from build123d import *

# Parameters (mm, degrees)
BOSS_EXTRUDE1_DEPTH = 15
CUT_EXTRUDE1_DEPTH  = 1.5
SKETCH3_R           = 1.75
CUT_EXTRUDE2_DEPTH  = 9.5
SKETCH5_W           = 31
SKETCH5_H           = 4
CUT_EXTRUDE3_DEPTH  = 54.5
SKETCH9_R           = 5.75
CUT_EXTRUDE6_DEPTH  = 30
CUT_EXTRUDE7_DEPTH  = 1
CUT_EXTRUDE8_DEPTH  = 36


with BuildPart() as part:
    # Sketch1 → Boss-Extrude1 (new body)
    with BuildSketch(Plane.XY):
        with BuildLine():
            Line((0, 20), (40, 20))
            Line((40, 20), (40, -20))
            Line((40, -20), (0, -20))
            ThreePointArc((0, -20), (-20, 0), (0, 20))
        make_face()
    extrude(amount=BOSS_EXTRUDE1_DEPTH)

    # Sketch2 → Cut-Extrude1 (cut)
    with BuildSketch(Plane.XY.offset(15)):
        Polygon((0, 3.58), (-3.100370946, 1.79), (-3.100370946, -1.79), (0, -3.58), (3.100370946, -1.79), (3.100370946, 1.79), align=None)
    cut_extrude1 = extrude(amount=-CUT_EXTRUDE1_DEPTH, mode=Mode.SUBTRACT)

    # Mirror1: Cut-Extrude1 across plane
    add(cut_extrude1.mirror(Plane.XY.offset(7.5)), mode=Mode.SUBTRACT)

    # Sketch3 → Cut-Extrude2 (cut)
    with BuildSketch(Plane.XY.offset(13.5)):
        Circle(SKETCH3_R)
    extrude(amount=-CUT_EXTRUDE2_DEPTH, mode=Mode.SUBTRACT)

    # Sketch5 → Cut-Extrude3 (cut)
    with BuildSketch(Plane.XZ.offset(20)):
        with Locations((-4.5, 7.5)):
            Rectangle(SKETCH5_W, SKETCH5_H)
    extrude(amount=-CUT_EXTRUDE3_DEPTH, mode=Mode.SUBTRACT)

    # Loft2: read off the stored shape, not the designer's step
    # Loft2: loft between two sections, ruled curve by curve
    loft2_from = [
        Edge.make_bspline([(60, 9.363291776, 3.988765584), (60, 9.089319173, 3.258171977), (60, 8.706678231, 2.497933469), (60, 7.661601681, 1.009485762), (60, 6.997280046, 0.281867871), (60, 5.377038752, -0.99416351), (60, 4.420018042, -1.539958552), (60, 2.836034453, -2.105793102), (60, 2.284258254, -2.252472584), (60, 1.154936709, -2.449606951), (60, 0.57750039, -2.5), (60, -0.57750039, -2.5), (60, -1.154936709, -2.449606951), (60, -2.284258254, -2.252472584), (60, -2.836034453, -2.105793102), (60, -4.420018042, -1.539958552), (60, -5.377038752, -0.99416351), (60, -6.997280046, 0.281867871), (60, -7.661601681, 1.009485762), (60, -8.706678231, 2.497933469), (60, -9.089319173, 3.258171977), (60, -9.363291776, 3.988765584)], [0, 0, 0, 0, 0.125, 0.125, 0.25, 0.25, 0.375, 0.375, 0.4375, 0.4375, 0.5, 0.5, 0.5625, 0.5625, 0.625, 0.625, 0.75, 0.75, 0.875, 0.875, 1, 1, 1, 1], 3),
        Edge.make_bspline([(60, -9.363291776, 3.988765584), (60, -9.568771228, 4.53671079), (60, -9.729102032, 5.111695552), (60, -9.944756725, 6.291183156), (60, -10, 6.895551394), (60, -10, 8.104448606), (60, -9.944756725, 8.708816844), (60, -9.729102032, 9.888304448), (60, -9.568771228, 10.46328921), (60, -9.363291776, 11.011234416)], [0, 0, 0, 0, 0.25, 0.25, 0.5, 0.5, 0.75, 0.75, 1, 1, 1, 1], 3),
        Edge.make_bspline([(60, 9.363291776, 11.011234416), (60, 9.568771228, 10.46328921), (60, 9.729102032, 9.888304448), (60, 9.944756725, 8.708816844), (60, 10, 8.104448606), (60, 10, 6.895551394), (60, 9.944756725, 6.291183156), (60, 9.729102032, 5.111695552), (60, 9.568771228, 4.53671079), (60, 9.363291776, 3.988765584)], [0, 0, 0, 0, 0.25, 0.25, 0.5, 0.5, 0.75, 0.75, 1, 1, 1, 1], 3),
        Edge.make_bspline([(60, -9.363291776, 11.011234416), (60, -9.089319173, 11.741828023), (60, -8.706678231, 12.502066531), (60, -7.661601681, 13.990514238), (60, -6.997280046, 14.718132129), (60, -5.377038752, 15.99416351), (60, -4.420018042, 16.539958552), (60, -2.836034453, 17.105793102), (60, -2.284258254, 17.252472584), (60, -1.154936709, 17.449606951), (60, -0.57750039, 17.5), (60, 0.57750039, 17.5), (60, 1.154936709, 17.449606951), (60, 2.284258254, 17.252472584), (60, 2.836034453, 17.105793102), (60, 4.420018042, 16.539958552), (60, 5.377038752, 15.99416351), (60, 6.997280046, 14.718132129), (60, 7.661601681, 13.990514238), (60, 8.706678231, 12.502066531), (60, 9.089319173, 11.741828023), (60, 9.363291776, 11.011234416)], [0, 0, 0, 0, 0.125, 0.125, 0.25, 0.25, 0.375, 0.375, 0.4375, 0.4375, 0.5, 0.5, 0.5625, 0.5625, 0.625, 0.625, 0.75, 0.75, 0.875, 0.875, 1, 1, 1, 1], 3),
    ]
    loft2_to = [
        Edge.make_bspline([(40, 20, 0), (40, 18.333333333, 0), (40, 16.666666667, 0), (40, 13.333333333, 0), (40, 11.666666667, 0), (40, 8.333333333, 0), (40, 6.666666667, 0), (40, 4.166666667, 0), (40, 3.333333333, 0), (40, 1.666666667, 0), (40, 0.833333333, 0), (40, -0.833333333, 0), (40, -1.666666667, 0), (40, -3.333333333, 0), (40, -4.166666667, 0), (40, -6.666666667, 0), (40, -8.333333333, 0), (40, -11.666666667, 0), (40, -13.333333333, 0), (40, -16.666666667, 0), (40, -18.333333333, 0), (40, -20, 0)], [0, 0, 0, 0, 0.125, 0.125, 0.25, 0.25, 0.375, 0.375, 0.4375, 0.4375, 0.5, 0.5, 0.5625, 0.5625, 0.625, 0.625, 0.75, 0.75, 0.875, 0.875, 1, 1, 1, 1], 3),
        Edge.make_bspline([(40, -20, 0), (40, -20, 1.25), (40, -20, 2.5), (40, -20, 5), (40, -20, 6.25), (40, -20, 8.75), (40, -20, 10), (40, -20, 12.5), (40, -20, 13.75), (40, -20, 15)], [0, 0, 0, 0, 0.25, 0.25, 0.5, 0.5, 0.75, 0.75, 1, 1, 1, 1], 3),
        Edge.make_bspline([(40, 20, 15), (40, 20, 13.75), (40, 20, 12.5), (40, 20, 10), (40, 20, 8.75), (40, 20, 6.25), (40, 20, 5), (40, 20, 2.5), (40, 20, 1.25), (40, 20, 0)], [0, 0, 0, 0, 0.25, 0.25, 0.5, 0.5, 0.75, 0.75, 1, 1, 1, 1], 3),
        Edge.make_bspline([(40, -20, 15), (40, -18.333333333, 15), (40, -16.666666667, 15), (40, -13.333333333, 15), (40, -11.666666667, 15), (40, -8.333333333, 15), (40, -6.666666667, 15), (40, -4.166666667, 15), (40, -3.333333333, 15), (40, -1.666666667, 15), (40, -0.833333333, 15), (40, 0.833333333, 15), (40, 1.666666667, 15), (40, 3.333333333, 15), (40, 4.166666667, 15), (40, 6.666666667, 15), (40, 8.333333333, 15), (40, 11.666666667, 15), (40, 13.333333333, 15), (40, 16.666666667, 15), (40, 18.333333333, 15), (40, 20, 15)], [0, 0, 0, 0, 0.125, 0.125, 0.25, 0.25, 0.375, 0.375, 0.4375, 0.4375, 0.5, 0.5, 0.5625, 0.5625, 0.625, 0.625, 0.75, 0.75, 0.875, 0.875, 1, 1, 1, 1], 3),
    ]
    loft2 = Solid(Shell([*[Face.make_surface_from_curves(loft2_from[k], loft2_to[k]) for k in range(4)], Face(Wire(loft2_from)), Face(Wire(loft2_to))]))
    add(loft2)

    # Sketch9 → Cut-Extrude6 (cut)
    with BuildSketch(Plane(origin=(60, 0, 0), x_dir=(0, 0, -1), z_dir=(1, 0, 0))):
        with Locations((-7.5, 0)):
            Circle(SKETCH9_R)
    extrude(amount=-CUT_EXTRUDE6_DEPTH, mode=Mode.SUBTRACT)

    # Sketch10 → Cut-Extrude7 (cut)
    with BuildSketch(Plane(origin=(0, 0, 0), x_dir=(-1, 0, 0), z_dir=(0, 0, -1))):
        Polygon((-34.996252953, 3.58), (-38.096623899, 1.79), (-38.096623899, -1.79), (-34.996252953, -3.58), (-31.895882008, -1.79), (-31.895882008, 1.79), align=None)
    cut_extrude7 = extrude(amount=-CUT_EXTRUDE7_DEPTH, mode=Mode.SUBTRACT)

    # Mirror4: Cut-Extrude7 across plane
    add(cut_extrude7.mirror(Plane.XY.offset(7.5)), mode=Mode.SUBTRACT)

    # Sketch11 → Cut-Extrude8 (cut)
    with BuildSketch(Plane(origin=(0, 0, 1), x_dir=(-1, 0, 0), z_dir=(0, 0, -1))):
        with BuildLine():
            ThreePointArc((-33.246252953, 0), (-33.758816086, 1.237436867), (-34.996252953, 1.75))
            Line((-34.996252953, 1.75), (-34.996252953, -1.75))
            ThreePointArc((-34.996252953, -1.75), (-33.758816086, -1.237436867), (-33.246252953, 0))
        make_face()
        with BuildLine():
            Line((-34.996252953, -1.75), (-34.996252953, 1.75))
            ThreePointArc((-34.996252953, 1.75), (-36.746252953, 0), (-34.996252953, -1.75))
        make_face()
    extrude(amount=-CUT_EXTRUDE8_DEPTH, mode=Mode.SUBTRACT)


solid = part.part
Can you work these out from the model? Positions are in its coordinate system, mm. A direction names the side the tool comes from. Coordinates: 2 decimals unless noted, no trailing zeros. Loops run counter-clockwise (first coordinate to the right, second up) from the corner with the lowest first, then second, coordinate; pieces in that order, holes last. Notation, with made-up numbers: (18, -34.5) - (53, -34.5) arc R33 ccw to (53, -2.5) - close; hole circle Ø9 at (-4, 61). An arc over 180 degrees is marked (long way). Answer as a JSON object with one key per item and string values. Group by question number.
Item 1: If I drill on L1, parallel to Z at x = -17, y = -9.5; L2, parallel to Y at x = 0, z = 4.95; L3, parallel to Z at x = 14.5, y = 11, over which ranges is the centre line in solid material (lowest first)? Write a range as from..to.
Item 2: If we section it at B-B (x = 15.5): List the corners of the cut face in (y, z) for me, plus the area to 3 significant figures.
Item 3: If we section it at A-A (x = 39): List the corners of the cut face in (y, z) for me.
Item 4: On a 3-axis mill with a long thin cutter (end or side, diameter ignored), from which of +Z, -Z, +X, -X, +Y, -Y can I reach the whole of each face in a straight line? I mean faces 4 (the face through (11, 0, 7)), 5 (the face through (-1.528, 2.698, 0.74)), 6 (the face through (10, 0, 0)), 7 (the face through (33.42, 2.67, 14.51)). Say none if no direction works.
Item 5: For pin 1 (7 mm diameter, centred on x = 35, y = 1, fed in from +Z); pin 2 (2 mm diameter, centred on x = 0, y = 0, fed in from +Z); pin 3 (5 mm diameter, centred on y = 5.5, z = 2.5, fed in from -X); pin 4 (8 mm diameter, centred on x = -1, z = 15.5, fed in from -Y), each with a flat end and sliding along its axis, tell me the tip position at first contact or that it passes through.
Item 6: If we mould it in two halves opening along Y, with no side actions, what happens to faces 1 (the face through (34, 2, 1)), 2 (the face through (10, 0, 15)), 3 (the face through (-20, 0, 3))? For each: released by +Y, released by -Y, zero draft, split by the parting line, or undercut.
Returned:
{
 "1": {"L1": "z = 0..5.5, 9.5..15", "L2": "y = -20..-1.75, 1.75..20", "L3": "z = 0..15"},
 "2": {"outline": "(-20, 0) - (20, 0) - (20, 15) - (-20, 15) - close", "area": "600 mm²"},
 "3": {"outline": "(-20, 0) - (20, 0) - (20, 15) - (-20, 15) - close; hole circle Ø11.5 at (0, 7.5)"},
 "4": {"face 4": "-X, +Y, -Y", "face 5": "-Z", "face 6": "-Z, -X, +Y, -Y", "face 7": "+Z"},
 "5": {"pin 1": "stops at z = 15", "pin 2": "stops at z = 4", "pin 3": "stops at x = -19.77", "pin 4": "stops at y = -20"},
 "6": {"face 1": "undercut", "face 2": "zero draft", "face 3": "split by the parting line"}
}
